from build123d import *

# Parameters (mm, degrees)
F0_W     = 72
F0_H     = 56
F0_R     = 5.5
F1_DEPTH = 3
F0_R_2   = 4
F2_DEPTH = 11.5
F3_DEPTH = 15


with BuildPart() as f1:
    # F0 (on Top) → F1 (new body)
    with BuildSketch(Plane.XY):
        with Locations((36, 28)):
            Rectangle(F0_W, F0_H)
        with Locations((13, 13)):
            Circle(F0_R, mode=Mode.SUBTRACT)
        with Locations((59, 13)):
            Circle(F0_R, mode=Mode.SUBTRACT)
        with Locations((13, 43)):
            Circle(F0_R, mode=Mode.SUBTRACT)
        with Locations((59, 43)):
            Circle(F0_R, mode=Mode.SUBTRACT)
    extrude(amount=F1_DEPTH)

    # F0 (on Top) → F2 (join)
    with BuildSketch(Plane.XY):
        with Locations((59, 13)):
            Circle(F0_R)
        with Locations((59, 13)):
            Circle(F0_R_2, mode=Mode.SUBTRACT)
        with Locations((59, 43)):
            Circle(F0_R)
        with Locations((59, 43)):
            Circle(F0_R_2, mode=Mode.SUBTRACT)
        with Locations((13, 43)):
            Circle(F0_R)
        with Locations((13, 43)):
            Circle(F0_R_2, mode=Mode.SUBTRACT)
        with Locations((13, 13)):
            Circle(F0_R)
        with Locations((13, 13)):
            Circle(F0_R_2, mode=Mode.SUBTRACT)
    extrude(amount=F2_DEPTH)

    # F0 (on Top) → F3 (join)
    with BuildSketch(Plane.XY):
        with Locations((13, 43)):
            Circle(F0_R_2)
        with Locations((59, 43)):
            Circle(F0_R_2)
        with Locations((59, 13)):
            Circle(F0_R_2)
        with Locations((13, 13)):
            Circle(F0_R_2)
    extrude(amount=F3_DEPTH)


solid = f1.part
The model under review builds one solid part; all positions refer to its coordinate system, in mm. A direction names the side the tool comes from. Give positions to 0.01 mm unless a question says otherwise; leave off trailing zeros. Write each loop counter-clockwise with the first axis right and the second up, starting at its lowest first coordinate (ties: lowest second). Pieces come first, ordered by that corner, then holes.
1. Add section D-D, the plane z = 9.75. Write out the cut boundary in (x, y), plus the area to 3 significant figures.
2. Draft analysis for pull direction Y (two halves, no side actions). For faces 3 (the cylindrical face through (10.05, 15.7, 13.23)), 4 (the flat face through (13, 13, 15)), 5 (the flat face through (35, 56, 1)), state which applies: +Y half, -Y half, draft (parallel to the pull), parting line (faces both ways), or undercut.
3. Wall thickness on L1, parallel to Y at x = 13, z = 9.5; L2, parallel to Z at x = 6, y = 45; L3, parallel to X at y = 15, z = 8.5: over which ranges is each line inside the solid? List them lowest first.
4. Add section A-A, the plane z = 14.25. Write out the cut boundary in (x, y).
5. Add section B-B, the plane y = 43. Write out the cut boundary in (x, z), plus the area to 3 significant figures.
6. For P1, Ø2, axis at x = 53, y = 15.5, coming from the -Z side; P2, Ø1, axis at y = 44, z = 11.5, coming from the -X side; P3, Ø2, axis at y = 21, z = 4.5, coming from the -X side, all flat-tipped, find the tip position at first contact; note any pin that passes through.
7. Tool access review of faces 1 (the flat face through (35, 28, 0)), 2 (the flat face through (55, 11, 11.5)): name each direction out of +Z, -Z, +X, -X, +Y, -Y from which nothing blocks a thin tool from reaching the whole face with its end or side.
8. Add section C-C, the plane x = 13. Write out the cut boundary in (y, z), plus the area to 3 significant figures.
Worked answers:
1. outline: circle Ø11 at (13, 13); circle Ø11 at (13, 43); circle Ø11 at (59, 13); circle Ø11 at (59, 43)
1. area: 380 mm2
2. face 3: undercut
2. face 4: draft
2. face 5: +Y half
3. L1: y = 7.5 to 18.5, 37.5 to 48.5
3. L2: z = 0 to 3
3. L3: x = 7.88 to 18.12, 53.88 to 64.12
4. outline: circle Ø8 at (13, 13); circle Ø8 at (13, 43); circle Ø8 at (59, 13); circle Ø8 at (59, 43)
5. outline: (0, 0) - (72, 0) - (72, 3) - (64.5, 3) - (64.5, 11.5) - (63, 11.5) - (63, 15) - (55, 15) - (55, 11.5) - (53.5, 11.5) - (53.5, 3) - (18.5, 3) - (18.5, 11.5) - (17, 11.5) - (17, 15) - (9, 15) - (9, 11.5) - (7.5, 11.5) - (7.5, 3) - (0, 3) - close
5. area: 459 mm2
6. P1: stops at z = 0
6. P2: stops at x = 7.52
6. P3: passes through
7. face 1: -Z, +X, -X, +Y, -Y
7. face 2: +Z
8. outline: (0, 0) - (56, 0) - (56, 3) - (48.5, 3) - (48.5, 11.5) - (47, 11.5) - (47, 15) - (39, 15) - (39, 11.5) - (37.5, 11.5) - (37.5, 3) - (18.5, 3) - (18.5, 11.5) - (17, 11.5) - (17, 15) - (9, 15) - (9, 11.5) - (7.5, 11.5) - (7.5, 3) - (0, 3) - close
8. area: 411 mm2
